Geometry: see drawing. Coordinates: mm, zero at the bounding-box minimum. A direction names the side the tool comes from. Round coordinates to 2 decimals unless told otherwise and drop trailing zeros. Loops run counter-clockwise (first coordinate to the right, second up) from the corner with the lowest first, then second, coordinate; pieces in that order, holes last. Notation, with made-up numbers: (-25.75, -1) - (-13.75, -1) arc R12 ccw to (-13.75, 21) - close; hole circle Ø7 at (-3, -40). An arc over 180 degrees is marked (long way). Use CSV: the item, a comma, the result in double quotes. Start each with the question number.
1. Pull-direction query (X, two-part tool) for the marked faces 1, 2 and 3; classes: +X half, -X half, draft (parallel to the pull), parting line (faces both ways), or undercut.
2. Pin query (flat end, axial travel): P1, Ø3.5, axis at x = 24, z = 11, coming from the -Y side; P2, Ø2, axis at y = 12.5, z = 11, coming from the -X side; P3, Ø1.5, axis at x = 19, y = 12, coming from the +Z side. Return the tip coordinate at first contact, or that it passes through.
3. Cut plane B-B (x = 34.5). Return loops of the section in (y, z), and give its area (4 significant figures).
4. Access query for the marked faces 4, 5 and 6. Directions: +Z, -Z, +X, -X, +Y, -Y. A direction counts if a zero-diameter tool reaches every point of the face in a straight line with its end or side. Return the directions, or none.
5. Cut plane D-D (z = 8.75). Return loops of the section in (x, y), and give its area (3 significant figures).
6. Cut plane A-A (z = 4.75). Return loops of the section in (x, y).
7. Material intervals for probe 1 along Y at (x, z) = (8, 6.5); probe 2 along Y at (x, z) = (28.5, 13.5); probe 3 along X at (y, z) = (6, 5.25), sorted ascending. Write a range as from..to.
8. Cut plane C-C (y = 13). Return loops of the section in (x, z), and give its area (4 significant figures).
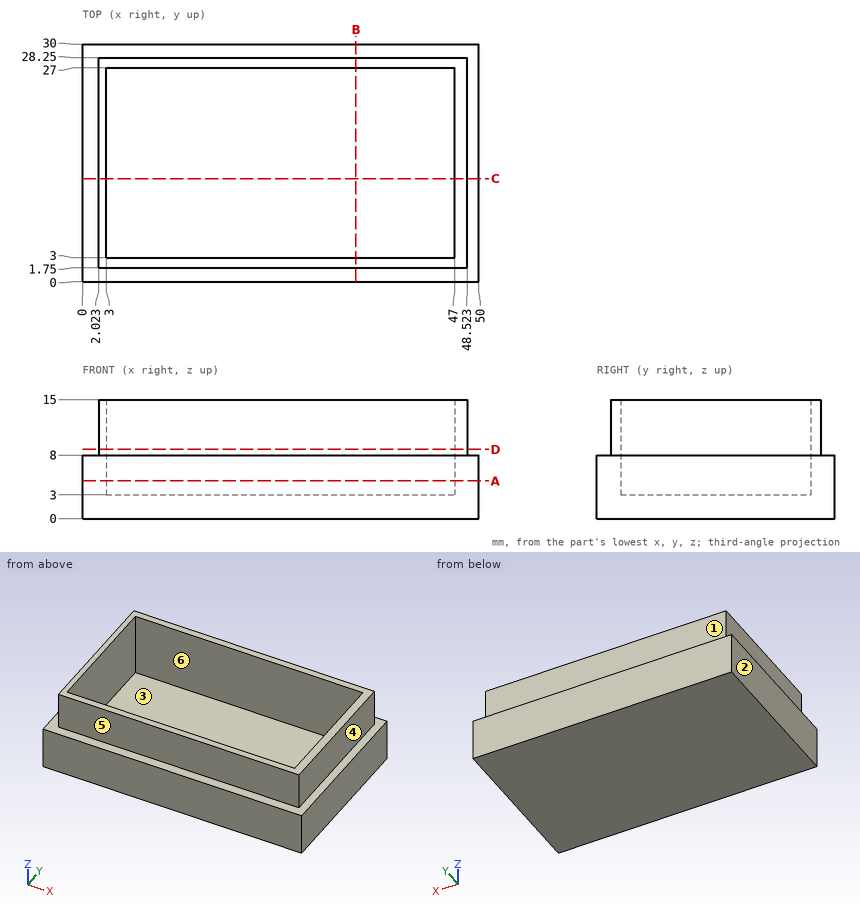
Established:
1,face 1,"draft"
1,face 2,"-X half"
1,face 3,"undercut"
2,P1,"stops at y = 1.75"
2,P2,"stops at x = 2.02"
2,P3,"stops at z = 3"
3,outline,"(0, 0) - (30, 0) - (30, 8) - (28.25, 8) - (28.25, 15) - (27, 15) - (27, 3) - (3, 3) - (3, 15) - (1.75, 15) - (1.75, 8) - (0, 8) - close"
3,area,"137.5 mm2"
4,face 4,"+Z, +X, +Y, -Y"
4,face 5,"+Z, +X, -X, -Y"
4,face 6,"+Z"
5,outline,"(2.02, 1.75) - (48.52, 1.75) - (48.52, 28.25) - (2.02, 28.25) - close; hole (3, 3) - (47, 3) - (47, 27) - (3, 27) - close"
5,area,"176 mm2"
6,outline,"(0, 0) - (50, 0) - (50, 30) - (0, 30) - close; hole (3, 3) - (47, 3) - (47, 27) - (3, 27) - close"
7,probe 1,"y = 0..3, 27..30"
7,probe 2,"y = 1.75..3, 27..28.25"
7,probe 3,"x = 0..3, 47..50"
8,outline,"(0, 0) - (50, 0) - (50, 8) - (48.52, 8) - (48.52, 15) - (47, 15) - (47, 3) - (3, 3) - (3, 15) - (2.02, 15) - (2.02, 8) - (0, 8) - close"
8,area,"197.5 mm2"
